Check sheet for the drawn part. Datum: minimum x, y, z corner. Units: mm. Give positions to 0.01 mm unless a question says otherwise; leave off trailing zeros. Loops run counter-clockwise (first coordinate to the right, second up) from the corner with the lowest first, then second, coordinate; pieces in that order, holes last.
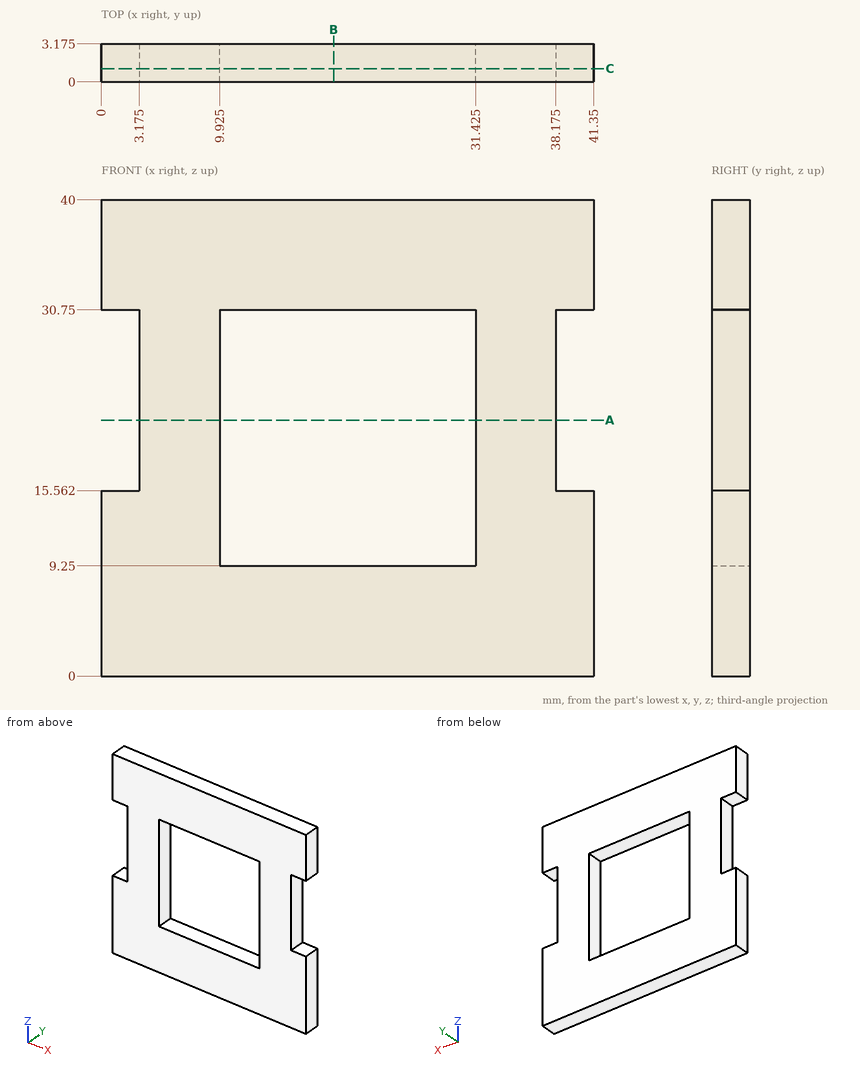
(1) Section check C-C on y = 1.1. Record the boundary of the cut face in (x, z) (3 decimals).
(2) Material ranges on line 1 (X direction, y = 0.95, z = 26.5) (3 decimals); line 2 (Z direction, x = 27.5, y = 2.8); line 3 (X direction, y = 1.9, z = 14.5) (3 decimals), recorded low to high.
(3) Section check B-B on x = 19.5. Record the boundary of the cut face in (y, z) (3 decimals).
(4) Section check A-A on z = 21.5. Record the boundary of the cut face in (x, y) (3 decimals).
(5) Gauge pin test, flat end, axial feed: pin 1 Ø1.6 at (y, z) = (1.5, 27) entering from -X (3 decimals). Record the tip position at first contact, or that the pin passes through.
Computed values:
1. outline: (0, 0) - (41.35, 0) - (41.35, 15.562) - (38.175, 15.562) - (38.175, 30.75) - (41.35, 30.75) - (41.35, 40) - (0, 40) - (0, 30.75) - (3.175, 30.75) - (3.175, 15.562) - (0, 15.562) - close; hole (9.925, 9.25) - (31.425, 9.25) - (31.425, 30.75) - (9.925, 30.75) - close
2. line 1: x = 3.175 to 9.925, 31.425 to 38.175
2. line 2: z = 0 to 9.25, 30.75 to 40
2. line 3: x = 0 to 9.925, 31.425 to 41.35
3. outline: (0, 0) - (3.175, 0) - (3.175, 9.25) - (0, 9.25) - close; (0, 30.75) - (3.175, 30.75) - (3.175, 40) - (0, 40) - close
4. outline: (3.175, 0) - (9.925, 0) - (9.925, 3.175) - (3.175, 3.175) - close; (31.425, 0) - (38.175, 0) - (38.175, 3.175) - (31.425, 3.175) - close
5. pin 1: stops at x = 3.175
